Geometry check sheet. Reference: the model listing, model coordinates, mm. A direction names the side the tool comes from. Coordinates: 2 decimals unless noted, no trailing zeros. Loops run counter-clockwise (first coordinate to the right, second up) from the corner with the lowest first, then second, coordinate; pieces in that order, holes last. Notation, with made-up numbers: (84.5, 41) - (108.5, 41) arc R25 cw to (108.5, 60) - close; hole circle Ø7 at (87.25, 7). An arc over 180 degrees is marked (long way). One line per item, written item: value.
Autodesk Inventor part; units mm, degrees
ref_plane "YZ Plane" through (0, 0, 0) normal (1, 0, 0) x (0, 1, 0)
ref_plane "XZ Plane" through (0, 0, 0) normal (0, 1, 0) x (-1, 0, 0)
ref_plane "XY Plane" through (0, 0, 0) normal (0, 0, 1) x (1, 0, 0)
sketch "Sketch1" plane through (0, 0, 0) normal (0, 1, 0) x (-1, 0, 0)
  line L0 (-20.5, 10.5) -> (20.5, 10.5)
  line L1 (20.5, 10.5) -> (20.5, -10.5)
  line L2 (20.5, -10.5) -> (-20.5, -10.5)
  line L3 (-20.5, -10.5) -> (-20.5, 10.5)
  line L4 (-20.5, 10.5) -> (20.5, -10.5) construction
  line L5 (20.5, 10.5) -> (-20.5, -10.5) construction
  line L6 (20.5, 10.5) -> (28.5, 10.5)
  line L7 (28.5, 10.5) -> (28.5, -30.5)
  line L8 (28.5, -30.5) -> (-28.5, -30.5)
  line L9 (-28.5, -30.5) -> (-28.5, 10.5)
  line L10 (-28.5, 10.5) -> (-20.5, 10.5)
  line L11 (-25.25, -5) -> (25.25, -5) construction
  line L12 (25.25, -5) -> (25.25, 5) construction
  line L13 (25.25, 5) -> (-25.25, 5) construction
  line L14 (-25.25, 5) -> (-25.25, -5) construction
  line L15 (-25.25, -5) -> (25.25, 5) construction
  line L16 (25.25, -5) -> (-25.25, 5) construction
  point P0 (0, 0)
  dimension "d0" = 41
  dimension "d1" = 21
  dimension "d2" = 8
  dimension "d3" = 41
  dimension "d4" = 8
  dimension "d5" = 50.5
  dimension "d6" = 10
extrude "Extrusion1" add sketch "Sketch1" along normal blind 10 contours L3 L2 L1 L6 L7 L8 L9 L10
hole "Hole1" at (-25.25, 0, 5) at (-25.25, 0, -5) at (25.25, 0, 5) at (25.25, 0, -5) direction (0, 1, 0) diameter 2.5 end through all both
sketch "Sketch2" plane through (0, 10, 0) normal (0, 1, 0) x (1, 0, 0)
  line L0 (-28.5, 30.5) -> (-28.5, -10.5)
  line L1 (28.5, -10.5) -> (28.5, 30.5)
  line L2 (-28.5, 30.5) -> (28.5, 30.5)
  line L3 (28.5, 30.5) -> (28.5, 28.5)
  line L4 (28.5, 28.5) -> (-28.5, 28.5)
  line L5 (-28.5, 28.5) -> (-28.5, 30.5)
  point P0 (0, 0)
  dimension "d16" = 2
extrude "Extrusion2" add sketch "Sketch2" along normal blind 30
sketch "Sketch3" plane through (28.5, 0, 10.5) normal (1, 0, 0) x (0, 0, -1)
  line L0 (39, 10) -> (39, 40)
  line L1 (41.007, 0) -> (39, 0)
  line L2 (39, 0) -> (39, 40)
  line L3 (39, 40) -> (41.007, 40)
  line L4 (41.007, 40) -> (41.007, 0)
  point P0 (10.5, 0)
extrude "Extrusion3" add sketch "Sketch3" along normal blind 30
fillet "Fillet2" radius 10 2 edges at (28.5, 5, -28.5) (0, 10, -28.5)
fillet "Fillet2" radius 2 6 edges at (58.5, 40, -29.5035) (-28.5, 40, -29.5) (28.5, 5, 10.5) (20.5, 5, 10.5) (-20.5, 5, 10.5) (-28.5, 5, 10.5)
equation "\"d4\" = d2"
properties part number "servoholder"
(1) Cross-section at C-C on y = 9. State how many separate pieces and enclosed holes the cut face has, and give its area (3 significant figures).
Reply:
separate pieces: 1
enclosed holes: 4
area: 1,530 mm2
(2) Cross-section at A-A on z = 5. Record the cut outline in (x, y), and give its area (3 significant figures).
Reply:
outline: (-28.5, 0) - (-26.5, 0) - (-26.5, 10) - (-28.5, 10) - close; (-24, 0) - (-20.5, 0) - (-20.5, 10) - (-24, 10) - close; (20.5, 0) - (24, 0) - (24, 10) - (20.5, 10) - close; (26.5, 0) - (28.5, 0) - (28.5, 10) - (26.5, 10) - close
area: 110 mm2
(3) Go/stop test with flat-tipped pins: pin 1 Ø3 at (x, y) = (10, 2.5) entering from +Z; pin 2 Ø3 at (x, z) = (-25.25, -5) entering from +Y; pin 3 Ø3 at (x, y) = (-9, 4.5) entering from -Z. Record where each tip stops, or that it passes through.
Reply:
pin 1: z = -10.5
pin 2: y = 10
pin 3: z = -30.5
(4) Cross-section at D-D on x = -9. Record the cut outline in (y, z).
Reply:
outline: (0, -30.5) - (40, -30.5) - (40, -28.5) - (20, -28.5) arc R10 cw to (10, -18.5) - (10, -10.5) - (0, -10.5) - close
(5) Cross-section at B-B on x = 25.25. Record the cut outline in (y, z).
Reply:
outline: (0, -30.5) - (40, -30.5) - (40, -28.5) - (20, -28.5) arc R10 cw to (10, -18.5) - (10, -6.25) - (0, -6.25) - close; (0, -3.75) - (10, -3.75) - (10, 3.75) - (0, 3.75) - close; (0, 6.25) - (10, 6.25) - (10, 10.5) - (0, 10.5) - close
(6) Access from +Z, -Z, +X, -X, +Y, -Y to the whole of each face (thin tool, end or side, straight path). Record for faces 5 (the face through (24, 29, -28.5)), 6 (the face through (28.5, 5, -5)), 7 (the face through (-21.1, 5.07, 9.93)).
Reply:
face 5: +Z, +X, +Y
face 6: +Z, +X, +Y, -Y
face 7: +Z, +Y, -Y
(7) Material ranges on probe 1 along X at (y, z) = (7.25, 5); probe 2 along Z at (x, y) = (25.25, 3.25); probe 3 along X at (y, z) = (3.5, -10), recorded low to high. Write a range as from..to.
Reply:
probe 1: -28.5..-26.5, -24..-20.5, 20.5..24, 26.5..28.5
probe 2: -30.5..-6.25, -3.75..3.75, 6.25..10.5
probe 3: -28.5..-20.5, 20.5..28.5
(8) Release check for a two-part mould opening along X. For faces 1 (the face through (26.47, 5.07, -4.73)), 2 (the face through (43, 20, -30.507)), 3 (the face through (20.5, 5, -1)), 4 (the face through (-28.5, 8, -14)) record: pulls with the +X half, pulls with the -X half, needs draft (parallel to the pull), parting line crosses it, or undercut.
Reply:
face 1: undercut
face 2: needs draft
face 3: undercut
face 4: pulls with the -X half
